```python
from build123d import *
from OCP.BRepFilletAPI import BRepFilletAPI_MakeChamfer

# Parameters (mm, degrees)
SKETCH1_W               = 38
SKETCH1_H               = 120
SKETCH1_W_2             = 21
SKETCH1_H_2             = 41
BOSS_EXTRUDE1_DEPTH     = 11
SKETCH3_R               = 1.3
CUT_EXTRUDE1_DEPTH      = 8
FILLET3_R               = 19
BOSS_EXTRUDE2_DEPTH     = 8
CUT_EXTRUDE2_DEPTH      = 66.741919656
CUT_EXTRUDE2_DEPTH_BACK = 66.741919656
SKETCH7_W               = 32
SKETCH7_H               = 49
BOSS_EXTRUDE4_DEPTH     = 8
SKETCH8_W               = 38
SKETCH8_H               = 52
BOSS_EXTRUDE5_DEPTH     = 8
BOSS_EXTRUDE6_START     = 2
SKETCH24_R              = 9
BOSS_EXTRUDE6_DEPTH     = 2
FILLET4_R               = 16
SKETCH26_W              = 38
SKETCH26_H              = 27
CUT_EXTRUDE4_DEPTH      = 5
SKETCH27_W              = 13
SKETCH27_H              = 31
CUT_EXTRUDE5_DEPTH      = 74.518705262
SKETCH29_W              = 23
SKETCH29_H              = 13
CUT_EXTRUDE7_DEPTH      = 8
SKETCH28_R              = 6.5
CUT_EXTRUDE8_DEPTH      = 2
SKETCH30_W              = 6
SKETCH30_H              = 5
CUT_EXTRUDE9_DEPTH      = 20
CHAMFER3_SIZE           = 6
CHAMFER3_SIZE_2         = 20
FILLET6_R               = 8
FILLET7_R               = 6
FILLET10_R              = 2.5
SKETCH31_R              = 1.1
CUT_EXTRUDE10_DEPTH     = 8
SKETCH32_R              = 1.1
CUT_EXTRUDE11_DEPTH     = 8
CUT_EXTRUDE13_DEPTH     = 69.483574828
FILLET11_R              = 6
SKETCH35_R              = 16.875
SKETCH35_R_2            = 12.975
BOSS_EXTRUDE7_DEPTH     = 9
CUT_EXTRUDE14_DEPTH     = 1


# Some blends are built 0.0001 mm under size
with BuildPart() as part:
    # Sketch1 → Boss-Extrude1 (new body)
    with BuildSketch(Plane.XY):
        Rectangle(SKETCH1_W, SKETCH1_H)
        with Locations((0, -24.5)):
            Rectangle(SKETCH1_W_2, SKETCH1_H_2, mode=Mode.SUBTRACT)
    extrude(amount=BOSS_EXTRUDE1_DEPTH)

    # Sketch3 → Cut-Extrude1 (cut)
    with BuildSketch(Plane.XY.offset(10)):
        with Locations((-5, -0.5)):
            Circle(SKETCH3_R)
        with Locations((5, -0.5)):
            Circle(SKETCH3_R)
        with Locations((5, -48.5)):
            Circle(SKETCH3_R)
        with Locations((-5, -48.5)):
            Circle(SKETCH3_R)
    extrude(amount=-CUT_EXTRUDE1_DEPTH, mode=Mode.SUBTRACT)

    # Fillet3
    fillet3_edges = [part.edges().sort_by_distance(p)[0] for p in [
        (19, -60, 5.5),
        (-19, -60, 5.5),
    ]]
    fillet(fillet3_edges, radius=FILLET3_R - 0.0001)  # a hair under: the kernel refuses the full size

    # Sketch4 → Boss-Extrude2 (add)
    with BuildSketch(Plane.XY.offset(11)):
        with BuildLine():
            Line((19, -41), (19, 60))
            Line((19, 60), (-19, 60))
            Line((-19, 60), (-19, -41))
            ThreePointArc((-19, -41), (-13.435028843, -54.435028843), (0, -60))
            ThreePointArc((0, -60), (13.435028843, -54.435028843), (19, -41))
        make_face()
        with BuildLine():
            Line((16, -41), (16, 57))
            Line((16, 57), (-16, 57))
            Line((-16, 57), (-16, -41))
            ThreePointArc((-16, -41), (-11.313708499, -52.313708499), (0, -57))
            ThreePointArc((0, -57), (11.313708499, -52.313708499), (16, -41))
        make_face(mode=Mode.SUBTRACT)
    extrude(amount=BOSS_EXTRUDE2_DEPTH)

    # Sketch6 → Cut-Extrude2 (cut, two sides: drawn at the far end of the back side and taken through both)
    with BuildSketch(Plane(origin=(0, 0, 0), x_dir=(0, 0, -1), z_dir=(1, 0, 0)).offset(-CUT_EXTRUDE2_DEPTH_BACK)):
        with BuildLine():
            Line((-19, -60), (-13, -60))
            Line((-13, -60), (-17, -35))
            Line((-17, -35), (-17.230341833, -33.272436255))
            add(Edge.make_bspline(
                [(-19, -20), (-18.961218666, -24.506149192), (-18.200739257, -28.905127919), (-17.230341833, -33.272436255)],
                knots=[0, 0, 0, 0, 0.330908527, 0.330908527, 0.330908527, 0.330908527], degree=3))
            Line((-19, -20), (-19, -60))
        make_face()
        with BuildLine():
            Line((-17, -35), (-13, -60))
            add(Edge.make_bspline(
                [(-17.230341833, -33.272436255), (-15.268214572, -42.103060212), (-12.44785515, -50.804202435), (-13, -60)],
                knots=[0.330908527, 0.330908527, 0.330908527, 0.330908527, 1, 1, 1, 1], degree=3))
            Line((-17.230341833, -33.272436255), (-17, -35))
        make_face()
    extrude(amount=CUT_EXTRUDE2_DEPTH + CUT_EXTRUDE2_DEPTH_BACK, mode=Mode.SUBTRACT)

    # Sketch7 → Boss-Extrude4 (add)
    with BuildSketch(Plane.XY.offset(11)):
        with Locations((0, 32.5)):
            Rectangle(SKETCH7_W, SKETCH7_H)
    extrude(amount=BOSS_EXTRUDE4_DEPTH)

    # Sketch8 → Boss-Extrude5 (add)
    with BuildSketch(Plane(origin=(0, 0, 0), x_dir=(-1, 0, 0), z_dir=(0, 0, -1))):
        with Locations((0, 34)):
            Rectangle(SKETCH8_W, SKETCH8_H)
    extrude(amount=BOSS_EXTRUDE5_DEPTH)

    # Sketch24 → Boss-Extrude6 (add)
    with BuildSketch(Plane(origin=(0, 0, 0), x_dir=(-1, 0, 0), z_dir=(0, 0, -1)).offset(BOSS_EXTRUDE6_START)):
        with BuildLine():
            Line((-19, 8), (-19, -41))
            ThreePointArc((-19, -41), (-13.435028843, -54.435028843), (0, -60))
            ThreePointArc((0, -60), (13.435028843, -54.435028843), (19, -41))
            Line((19, -41), (19, 8))
            Line((19, 8), (-19, 8))
        make_face()
        with Locations((0, -34.75)):
            Circle(SKETCH24_R, mode=Mode.SUBTRACT)
    extrude(amount=-BOSS_EXTRUDE6_DEPTH)

    # Fillet4
    fillet4_edges = [part.edges().sort_by_distance(p)[0] for p in [
        (-16, 8, 15),
        (16, 8, 15),
    ]]
    fillet(fillet4_edges, radius=FILLET4_R - 0.0001)  # a hair under: the kernel refuses the full size

    # Sketch26 → Cut-Extrude4 (cut)
    with BuildSketch(Plane(origin=(0, 60, 0), x_dir=(1, 0, 0), z_dir=(0, 1, 0))):
        with Locations((0, -5.5)):
            Rectangle(SKETCH26_W, SKETCH26_H)
    extrude(amount=-CUT_EXTRUDE4_DEPTH, mode=Mode.SUBTRACT)

    # Sketch27 → Cut-Extrude5 (cut, through all)
    with BuildSketch(Plane(origin=(19, 0, 0), x_dir=(0, 0, -1), z_dir=(1, 0, 0))):
        with Locations((-5.5, 29.5)):
            Rectangle(SKETCH27_W, SKETCH27_H)
    extrude(amount=-CUT_EXTRUDE5_DEPTH, mode=Mode.SUBTRACT)

    # Sketch29 → Cut-Extrude7 (cut)
    with BuildSketch(Plane.XZ.offset(-45)):
        with Locations((0, 5.5)):
            Rectangle(SKETCH29_W, SKETCH29_H)
    extrude(amount=-CUT_EXTRUDE7_DEPTH, mode=Mode.SUBTRACT)

    # Sketch28 → Cut-Extrude8 (cut)
    with BuildSketch(Plane(origin=(0, 55, 0), x_dir=(1, 0, 0), z_dir=(0, 1, 0))):
        with Locations(Location((-5.3, -5.5, 0), (0, 0, 270))):
            Circle(SKETCH28_R)
    extrude(amount=-CUT_EXTRUDE8_DEPTH, mode=Mode.SUBTRACT)

    # Sketch30 → Cut-Extrude9 (cut)
    with BuildSketch(Plane(origin=(0, 14, 0), x_dir=(1, 0, 0), z_dir=(0, 1, 0))):
        with Locations((-16, -5.5)):
            Rectangle(SKETCH30_W, SKETCH30_H)
        with Locations((16, -5.5)):
            Rectangle(SKETCH30_W, SKETCH30_H)
    extrude(amount=-CUT_EXTRUDE9_DEPTH, mode=Mode.SUBTRACT)

    # Chamfer3
    chamfer3_edges_1 = [part.edges().sort_by_distance(p)[0] for p in [
        (13, -6, 5.5),
    ]]
    chamfer3_side_1 = [part.faces().sort_by_distance(p)[0] for p in [
        (13.12, -6, 5.5),
    ]]
    chamfer3_edges_2 = [part.edges().sort_by_distance(p)[0] for p in [
        (-13, -6, 5.5),
    ]]
    chamfer3_side_2 = [part.faces().sort_by_distance(p)[0] for p in [
        (-13.12, -6, 5.5),
    ]]
    chamfer3 = BRepFilletAPI_MakeChamfer(part.part.solid().wrapped)
    for e in chamfer3_edges_1:
        chamfer3.Add(CHAMFER3_SIZE - 0.0001, CHAMFER3_SIZE_2 - 0.0001, e.wrapped, chamfer3_side_1[0].wrapped)
    for e in chamfer3_edges_2:
        chamfer3.Add(CHAMFER3_SIZE - 0.0001, CHAMFER3_SIZE_2 - 0.0001, e.wrapped, chamfer3_side_2[0].wrapped)
    add(Compound.cast(chamfer3.Shape()), mode=Mode.REPLACE)  # a hair under: the kernel refuses the full size

    # Fillet6
    # the kernel refuses this fillet: 8 mm, written as the material it takes off along each edge
    with BuildSketch(Plane(origin=(-19, 14, -1), x_dir=(1, 0, 0), z_dir=(0, 0, 1))) as fillet6_piece_1_section:
        with BuildLine():
            CenterArc((FILLET6_R, -FILLET6_R), FILLET6_R, 90, 90)
            Line((0, -FILLET6_R), (0, 0))
            Line((0, 0), (FILLET6_R, 0))
        make_face()
    fillet6_piece_1 = extrude(amount=24, mode=Mode.PRIVATE)
    fillet6_piece_1 = split(fillet6_piece_1, bisect_by=Plane(origin=(-12.501601439, 13.924002019, 12), z_dir=(0, 0, -1)), keep=Keep.TOP, mode=Mode.PRIVATE)
    add(fillet6_piece_1, mode=Mode.SUBTRACT)
    with BuildSketch(Plane(origin=(19, 14, -1), x_dir=(-1, 0, 0), z_dir=(0, 0, 1))) as fillet6_piece_2_section:
        with BuildLine():
            CenterArc((FILLET6_R, FILLET6_R), FILLET6_R, 180, 90)
            Line((0, FILLET6_R), (0, 0))
            Line((0, 0), (FILLET6_R, 0))
        make_face()
    fillet6_piece_2 = extrude(amount=24, mode=Mode.PRIVATE)
    fillet6_piece_2 = split(fillet6_piece_2, bisect_by=Plane(origin=(12.501601439, 13.924002019, 12), z_dir=(0, 0, -1)), keep=Keep.TOP, mode=Mode.PRIVATE)
    add(fillet6_piece_2, mode=Mode.SUBTRACT)

    # Fillet7
    fillet7_edges = [part.edges().sort_by_distance(p)[0] for p in [
        (0, 8, -2),
    ]]
    fillet(fillet7_edges, radius=FILLET7_R - 0.0001)  # a hair under: the kernel refuses the full size

    # Fillet10
    fillet10_edges = [part.edges().sort_by_distance(p)[0] for p in [
        (16.041314475, 3.862066808, 3),
        (16.041314475, 3.862066808, 8),
        (-16.041314475, 3.862066808, 3),
        (-16.041314475, 3.862066808, 8),
    ]]
    fillet(fillet10_edges, radius=FILLET10_R - 0.0001)  # a hair under: the kernel refuses the full size

    # Sketch31 → Cut-Extrude10 (cut)
    with BuildSketch(Plane.XY.offset(11)):
        with Locations((-5, -0.5)):
            Circle(SKETCH31_R)
        with Locations((5, -0.5)):
            Circle(SKETCH31_R)
        with Locations((5, -48.5)):
            Circle(SKETCH31_R)
        with Locations((-5, -48.5)):
            Circle(SKETCH31_R)
    extrude(amount=-CUT_EXTRUDE10_DEPTH, mode=Mode.SUBTRACT)

    # Sketch32 → Cut-Extrude11 (cut)
    with BuildSketch(Plane.XZ.offset(-45)):
        with Locations(Location((13.8, 5.5, 0), (0, 0, 270))):
            Circle(SKETCH32_R)
        with Locations(Location((-13.8, 5.5, 0), (0, 0, 270))):
            Circle(SKETCH32_R)
    extrude(amount=-CUT_EXTRUDE11_DEPTH, mode=Mode.SUBTRACT)

    # Sketch34 → Cut-Extrude13 (cut, through all)
    with BuildSketch(Plane.XY.offset(19)):
        Polygon((16.5, 55), (19, 0), (19, 55), align=None)
        Polygon((-16.5, 55), (-19, 0), (-19, 55), align=None)
    extrude(amount=-CUT_EXTRUDE13_DEPTH, mode=Mode.SUBTRACT)

    # Fillet11
    # the kernel refuses this fillet: 6 mm, written as the material it takes off along each edge
    with BuildSketch(Plane(origin=(-20.271039429, -27.962867448, -8), x_dir=(0, 0, 1), z_dir=(0.04540766091865005, 0.9989685402102996, 0)), Plane(origin=(20.271039429, -27.962867448, -8), x_dir=(-0.9989685402102996, -0.04540766091865018, 0), z_dir=(-0.04540766091865018, 0.9989685402102996, 0))) as fillet11_piece_1:
        with BuildLine():
            CenterArc((FILLET11_R, FILLET11_R), FILLET11_R, 180, 90)
            Line((0, FILLET11_R), (-FILLET11_R * 0.02, FILLET11_R))
            Line((-FILLET11_R * 0.02, FILLET11_R), (-FILLET11_R * 0.02, -FILLET11_R * 0.02))
            Line((-FILLET11_R * 0.02, -FILLET11_R * 0.02), (FILLET11_R, -FILLET11_R * 0.02))
            Line((FILLET11_R, -FILLET11_R * 0.02), (FILLET11_R, 0))
        make_face()
    extrude(amount=119.048528665, mode=Mode.SUBTRACT)
    with BuildSketch(Plane(origin=(-14.865324207, 90.962867448, 19), x_dir=(0, 0, -1), z_dir=(-0.04540766091865005, -0.9989685402102996, 0)), Plane(origin=(14.865324207, 90.962867448, 19), x_dir=(-0.9989685402102996, -0.04540766091865018, 0), z_dir=(0.04540766091865018, -0.9989685402102996, 0))) as fillet11_piece_2:
        with BuildLine():
            CenterArc((FILLET11_R, FILLET11_R), FILLET11_R, 180, 90)
            Line((0, FILLET11_R), (-FILLET11_R * 0.02, FILLET11_R))
            Line((-FILLET11_R * 0.02, FILLET11_R), (-FILLET11_R * 0.02, -FILLET11_R * 0.02))
            Line((-FILLET11_R * 0.02, -FILLET11_R * 0.02), (FILLET11_R, -FILLET11_R * 0.02))
            Line((FILLET11_R, -FILLET11_R * 0.02), (FILLET11_R, 0))
        make_face()
    extrude(amount=127.056788864, mode=Mode.SUBTRACT)

    # Sketch35 → Boss-Extrude7 (add)
    with BuildSketch(Plane(origin=(0, 0, -2), x_dir=(-1, 0, 0), z_dir=(0, 0, -1))):
        with Locations((0, -34.75)):
            Circle(SKETCH35_R)
        with Locations((0, -34.75)):
            Circle(SKETCH35_R_2, mode=Mode.SUBTRACT)
    extrude(amount=BOSS_EXTRUDE7_DEPTH)

    # Sketch36 → Cut-Extrude14 (cut, symmetric)
    with BuildSketch(Plane(origin=(0, 0, 0), x_dir=(0, 0, -1), z_dir=(1, 0, 0))):
        Polygon((-11, -45), (-11, -53), (-8, -45), align=None)
        Polygon((-11, -4), (-11, 4), (-8, -4), align=None)
    extrude(amount=CUT_EXTRUDE14_DEPTH, both=True, mode=Mode.SUBTRACT)


solid = part.part
```
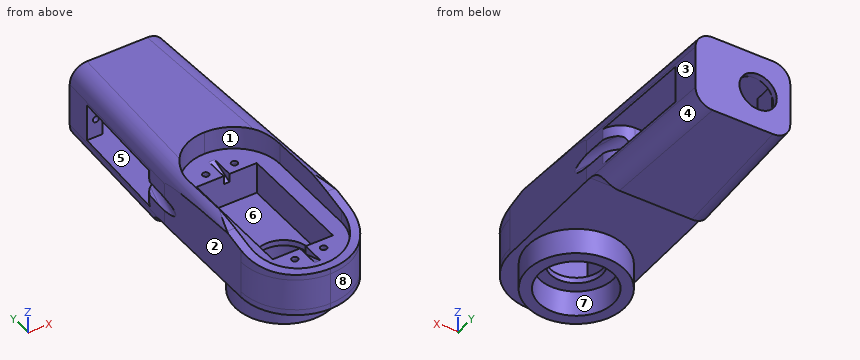
Source: CAD feature listing. Evaluate the final solid. Frame: model axes, mm. Face numbers are marked on the shaded views. A direction names the side the tool comes from. Give positions to 0.01 mm unless a question says otherwise; leave off trailing zeros. Loops run counter-clockwise (first coordinate to the right, second up) from the corner with the lowest first, then second, coordinate; pieces in that order, holes last. Notation, with made-up numbers: (-22, 33.25) - (-9, 33.25) arc R13 cw to (-9, 42.25) - close; hole circle Ø5 at (-23.5, -28.75). An arc over 180 degrees is marked (long way). Use CSV: the item, a comma, the result in double quotes. Start each with the question number.
1. Section A-A (z = 1). Count the separate pieces of the cut face and the enclosed holes in it, then the cut area to 3 significant figures.
2. Pin query (flat end, axial travel): pin 1 (2.5 mm diameter, centred on x = 15, z = 5, fed in from -Y); pin 2 (4 mm diameter, centred on x = 10.5, z = 3, fed in from -Y); pin 3 (17 mm diameter, centred on x = -4, y = -24.5, fed in from +Z). Return the tip coordinate at first contact, or that it passes through.
3. Reachability of the marked faces 4, 5, 6, 7 and 8 from +Z, -Z, +X, -X, +Y, -Y: full face, straight path, thin tool, end or side. Return the list, or none.
4. Draft query along Y for the marked faces 1, 2 and 3. Return one class per face: +Y half, -Y half, draft (parallel to the pull), parting line (faces both ways), or undercut.
5. Section B-B (z = -5.5). Output: boundary loops of the cut face in (x, y) (3 decimals), then the cut area to 3 significant figures.
6. Ray query, L1, parallel to Z at x = -10, y = 49; L2, parallel to Y at x = -5, z = 10.55; L3, parallel to Y at x = 5, z = 4.75. Return the intervals inside material, ascending.
Response:
1,separate pieces,"3"
1,enclosed holes,"1"
1,area,"1,900 mm²"
2,pin 1,"y = -54.11"
2,pin 2,"y = -57.99"
2,pin 3,"z = 11"
3,face 4,"-Z, +X, +Y"
3,face 5,"none"
3,face 6,"+Z"
3,face 7,"-Z"
3,face 8,"+Z, -Z, +X, -Y"
4,face 1,"undercut"
4,face 2,"draft"
4,face 3,"+Y half"
5,outline,"(-17.533, 7.454) - (17.533, 7.454) - (15.372, 55) - (-15.372, 55) - close; circle Ø33.75 at (0, -34.75); hole circle Ø25.95 at (0, -34.75)"
5,area,"1,930 mm²"
6,L1,"-8 to -1, 12 to 19"
6,L2,"-59.33 to -49.6, -47.4 to -45, -4 to -1.6, 0.6 to 14"
6,L3,"-59.33 to -49.8, -47.2 to -45, -4 to -1.8, 0.8 to 14, 53 to 55"
